Model file for the job. Use its own axes, mm. Round coordinates to 2 decimals unless told otherwise and drop trailing zeros. Loops run counter-clockwise (first coordinate to the right, second up) from the corner with the lowest first, then second, coordinate; pieces in that order, holes last. Notation, with made-up numbers: M -15.75,45 L 28.25,45 A36 cw 28.25,79 Z; hole C -16,17 d8. An arc over 180 degrees is marked long. Use a Markdown table: item, result. Add a question column.
Item 1: Wall check: L1, parallel to X at y = 42, z = 1.2; L2, parallel to Y at x = 40.5, z = 0.85; L3, parallel to X at y = 609.5, z = 2.55. Give the ranges that are in metal, low to high. Write a range as from..to.
Item 2: Saw through at C-C on y = 89. Write the cut outline in (x, z) (3 decimals).
Item 3: Pin check, flat tips, straight feed: P1, Ø1.6, axis at y = 674.5, z = 2.5, coming from the +X side; P2, Ø1.6, axis at x = 737.5, z = 2.5, coming from the -Y side; P3, Ø1.6, axis at x = 31.5, z = 1.5, coming from the +Y side. Stop position of each tip, or through.
Item 4: Saw through at B-B on x = 688.5. Write the cut outline in (y, z) (3 decimals), then the cut area to 3 significant figures.
```python
from build123d import *

# Parameters (mm, degrees)
SKETCH1_W           = 762
SKETCH1_H           = 711.2
BOSS_EXTRUDE1_DEPTH = 3.175
CUT_EXTRUDE1_DEPTH  = 4.175
FILLET1_R           = 3.175


with BuildPart() as part:
    # Sketch1 → Boss-Extrude1 (new body)
    with BuildSketch(Plane.XY):
        with Locations((381, 355.6)):
            Rectangle(SKETCH1_W, SKETCH1_H)
    extrude(amount=BOSS_EXTRUDE1_DEPTH)

    # Sketch2 → Cut-Extrude1 (cut, through all)
    with BuildSketch(Plane.XY.offset(3.175)):
        Polygon((0, 571.5), (50.8, 571.5), (139.7, 660.4), (139.7, 711.2), (0, 711.2), align=None)
        Polygon((139.7, 50.8), (139.7, 0), (0, 0), (0, 139.7), (50.8, 139.7), align=None)
        Polygon((762, 139.7), (711.2, 139.7), (622.3, 50.8), (622.3, 0), (762, 0), align=None)
        Polygon((622.3, 660.4), (622.3, 711.2), (762, 711.2), (762, 571.5), (711.2, 571.5), align=None)
    extrude(amount=-CUT_EXTRUDE1_DEPTH, mode=Mode.SUBTRACT)

    # Fillet1
    fillet1_edges = [part.edges().sort_by_distance(p)[0] for p in [
        (711.2, 571.5, 1.5875),
        (622.3, 660.4, 1.5875),
        (622.3, 711.2, 1.5875),
        (762, 571.5, 1.5875),
        (762, 139.7, 1.5875),
        (622.3, 0, 1.5875),
        (622.3, 50.8, 1.5875),
        (711.2, 139.7, 1.5875),
        (50.8, 139.7, 1.5875),
        (139.7, 50.8, 1.5875),
        (139.7, 0, 1.5875),
        (0, 139.7, 1.5875),
        (0, 571.5, 1.5875),
        (139.7, 711.2, 1.5875),
        (139.7, 660.4, 1.5875),
        (50.8, 571.5, 1.5875),
    ]]
    fillet(fillet1_edges, radius=FILLET1_R)


solid = part.part
```
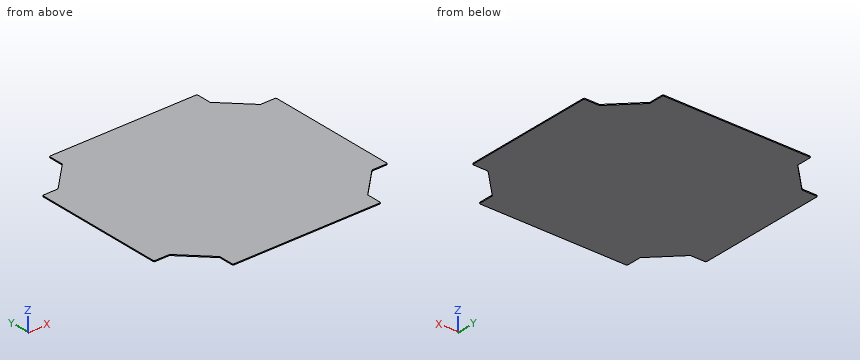
Entries:
| question | item | result |
|---|---|---|
| 1 | L1 | 139.7..622.3 |
| 1 | L2 | 139.7..571.5 |
| 1 | L3 | 88.8..673.2 |
| 2 | outline | M 101.5,0 L 660.5,0 L 660.5,3.175 L 101.5,3.175 Z |
| 3 | P1 | x = 622.3 |
| 3 | P2 | y = 139.7 |
| 3 | P3 | y = 571.5 |
| 4 | outline | M 117,0 L 594.2,0 L 594.2,3.175 L 117,3.175 Z |
| 4 | area | 1,520 mm2 |
